```python
from build123d import *

# Parameters (mm, degrees)
F0_R           = 2.5
F0_R_2         = 7.65
F1_DEPTH       = 5
F2_D           = 4.25
F2_CSINK_D     = 8
F2_CSINK_ANGLE = 90
F3_R           = 5


with BuildPart() as f1:
    # F0 (on Front) → F1 (new body)
    with BuildSketch(Plane.XZ):
        with BuildLine():
            Line((-15, 0), (0, 0))
            Line((0, 0), (15, 0))
            Line((15, 0), (15, 40))
            ThreePointArc((15, 40), (0, 55), (-15, 40))
            Line((-15, 40), (-15, 0))
        make_face()
        with Locations((0, 25.7251504809)):
            Circle(F0_R, mode=Mode.SUBTRACT)
        with Locations((0, 40)):
            Circle(F0_R_2, mode=Mode.SUBTRACT)
    extrude(amount=F1_DEPTH)

    # F2 (through all)
    with Locations(Plane(origin=(0, 0, 0), x_dir=(1, 0, 0), z_dir=(0, 1, 0))):
        with Locations((-7.5, -10), (7.5, -10)):
            CounterSinkHole(F2_D / 2, F2_CSINK_D / 2, counter_sink_angle=F2_CSINK_ANGLE)

    # F3
    f3_edges = [f1.edges().sort_by_distance(p)[0] for p in [
        (-15, -2.5, 0),
        (15, -2.5, 0),
    ]]
    fillet(f3_edges, radius=F3_R)


solid = f1.part
```
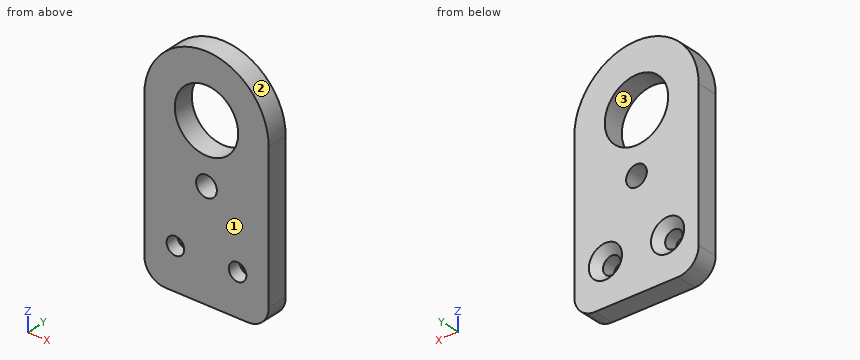
Input: part model. Units: mm. Frame: model coordinates. Face numbers are marked on the shaded views. Coordinates: 2 decimals unless noted, no trailing zeros. Loops run counter-clockwise (first coordinate to the right, second up) from the corner with the lowest first, then second, coordinate; pieces in that order, holes last. Notation, with made-up numbers: M 41,-12 L 83,-12 A24 cw 83,1 Z; hole C 76,31.5 d1. An arc over 180 degrees is marked long. Use a Markdown table: item, result. Add a question column.
1) Draft query along X for the marked faces 1, 2 and 3. Return one class per face: +X half, -X half, draft (parallel to the pull), parting line (faces both ways), or undercut.
2) Section B-B, the plane x = 0. Return the cut outline in (y, z), plus the area to 4 significant figures.
3) Section C-C, the plane y = -3.8. Return the cut outline in (x, z) (3 decimals), plus the area to 3 significant figures.
4) Section A-A, the plane z = 10. Return the cut outline in (x, y) (3 decimals), plus the area to 3 significant figures.
5) Section D-D, the plane z = 47. Return the cut outline in (x, y).
6) Line query: L1, parallel to Z at x = 0, y = -3.05; L2, parallel to Z at x = -1, y = -2.95; L3, parallel to Z at x = -10, y = -0.35. Output: solid intervals per line, ascending. Write a range as from..to.
Answer below:
| question | item | result |
|---|---|---|
| 1 | face 1 | draft |
| 1 | face 2 | parting line |
| 1 | face 3 | undercut |
| 2 | outline | M -5,0 L 0,0 L 0,23.23 L -5,23.23 Z; M -5,28.23 L 0,28.23 L 0,32.35 L -5,32.35 Z; M -5,47.65 L 0,47.65 L 0,55 L -5,55 Z |
| 2 | area | 173.5 mm2 |
| 3 | outline | M -15,5 A5 ccw -10,0 L 10,0 A5 ccw 15,5 L 15,40 A15 ccw -15,40 Z; hole C -7.5,10 d4.25; hole C 0,40 d15.3; hole C 0,25.725 d5; hole C 7.5,10 d4.25 |
| 3 | area | 1,310 mm2 |
| 4 | outline | M -15,-5 L -9.625,-5 L -9.625,-1.875 L -11.5,0 L -15,0 Z; M -5.375,-5 L 5.375,-5 L 5.375,-1.875 L 3.5,0 L -3.5,0 L -5.375,-1.875 Z; M 9.625,-5 L 15,-5 L 15,0 L 11.5,0 L 9.625,-1.875 Z |
| 4 | area | 100 mm2 |
| 5 | outline | M -13.27,-5 L -3.09,-5 L -3.09,0 L -13.27,0 Z; M 3.09,-5 L 13.27,-5 L 13.27,0 L 3.09,0 Z |
| 6 | L1 | 0..23.23, 28.23..32.35, 47.65..55 |
| 6 | L2 | 0..23.43, 28.02..32.42, 47.58..54.97 |
| 6 | L3 | 0..7.34, 12.66..51.18 |
